from build123d import *

# Parameters (mm, degrees)
SKETCH1_W                       = 49.784
SKETCH1_H                       = 35.56
BOSS_EXTRUDE1_DEPTH             = 50.8
M4X0_7_TAPPED_HOLE1_AT_2_COUNT  = 2
M4X0_7_TAPPED_HOLE1_AT_2_PITCH  = 30
M4X0_7_TAPPED_HOLE1_AT_3_COUNT  = 2
M4X0_7_TAPPED_HOLE1_AT_3_PITCH  = 18
M4X0_7_TAPPED_HOLE1_AT_4_COUNT  = 2
M4X0_7_TAPPED_HOLE1_AT_4_PITCH  = 24
CUT_EXTRUDE2_DEPTH              = 0.508
MIRROR2_START                   = -17.78
MIRROR2_DEPTH                   = 0.508
M5X0_8_TAPPED_HOLE1_D           = 4.2
M5X0_8_TAPPED_HOLE1_DEPTH       = 12.192
M5X0_8_TAPPED_HOLE1_CSINK_D     = 6
M5X0_8_TAPPED_HOLE1_CSINK_ANGLE = 90
M5X0_8_TAPPED_HOLE1_TIP         = 1.2618073


# Read off the part's stored shape, not the designer's step: Mirror2
with BuildPart() as part:
    # Sketch1 → Boss-Extrude1 (new body)
    with BuildSketch(Plane.YZ):
        Rectangle(SKETCH1_W, SKETCH1_H)
    extrude(amount=BOSS_EXTRUDE1_DEPTH)

    # Sketch3 → M4x0.7 Tapped Hole1 (revolve, cut)
    with BuildSketch(Plane(origin=(13.4, -24.892, -9), x_dir=(0, 0, -1), z_dir=(1, 0, 0))):
        Polygon((0, 0), (0, 10.897420021), (1.65, 9.906), (1.65, 0.85), (2.5, 0), align=None)
    m4x0_7_tapped_hole1 = revolve(axis=Axis((13.4, -31.242, -9), (0, 1, 0)), mode=Mode.SUBTRACT)

    # M4x0.7 Tapped Hole1 at 2: M4x0.7 Tapped Hole1 ×2
    with Locations(*[Vector(0.8000000000000002, 0, 0.5999999999999998) * (i * M4X0_7_TAPPED_HOLE1_AT_2_PITCH) for i in range(1, M4X0_7_TAPPED_HOLE1_AT_2_COUNT)]):
        add(m4x0_7_tapped_hole1, mode=Mode.SUBTRACT)

    # M4x0.7 Tapped Hole1 at 3: M4x0.7 Tapped Hole1 ×2
    with Locations(*[(0, 0, i * M4X0_7_TAPPED_HOLE1_AT_3_PITCH) for i in range(1, M4X0_7_TAPPED_HOLE1_AT_3_COUNT)]):
        add(m4x0_7_tapped_hole1, mode=Mode.SUBTRACT)

    # M4x0.7 Tapped Hole1 at 4: M4x0.7 Tapped Hole1 ×2
    with Locations(*[(i * M4X0_7_TAPPED_HOLE1_AT_4_PITCH, 0, 0) for i in range(1, M4X0_7_TAPPED_HOLE1_AT_4_COUNT)]):
        add(m4x0_7_tapped_hole1, mode=Mode.SUBTRACT)

    # Mirror1: M4x0.7 Tapped Hole1 across plane
    add(m4x0_7_tapped_hole1.mirror(Plane.ZX), mode=Mode.SUBTRACT)

    # Mirror1 copy 1 sketch → Mirror1 copy 1 (revolve, cut)
    with BuildSketch(Plane(origin=(37.4, 24.892, 9), x_dir=(0, 0, -1), z_dir=(1, 0, 0))):
        Polygon((0, 0), (0, -10.897420021), (1.65, -9.906), (1.65, -0.85), (2.5, 0), align=None)
    revolve(axis=Axis((37.4, 31.242, 9), (0, 1, 0)), mode=Mode.SUBTRACT)

    # Mirror1 copy 2 sketch → Mirror1 copy 2 (revolve, cut)
    with BuildSketch(Plane(origin=(13.4, 24.892, 9), x_dir=(0, 0, -1), z_dir=(1, 0, 0))):
        Polygon((0, 0), (0, -10.897420021), (1.65, -9.906), (1.65, -0.85), (2.5, 0), align=None)
    revolve(axis=Axis((13.4, 31.242, 9), (0, 1, 0)), mode=Mode.SUBTRACT)

    # Mirror1 copy 3 sketch → Mirror1 copy 3 (revolve, cut)
    with BuildSketch(Plane(origin=(37.4, 24.892, -9), x_dir=(0, 0, -1), z_dir=(1, 0, 0))):
        Polygon((0, 0), (0, -10.897420021), (1.65, -9.906), (1.65, -0.85), (2.5, 0), align=None)
    revolve(axis=Axis((37.4, 31.242, -9), (0, 1, 0)), mode=Mode.SUBTRACT)

    # Sketch5 → Cut-Revolve1 (revolve, cut)
    with BuildSketch(Plane(origin=(0, 0, 0), x_dir=(-1, 0, 0), z_dir=(0, 1, 0))):
        Polygon((-25.4, 17.78), (-25.4, 13.964535069), (-31.75, 17.78), align=None)
    revolve(axis=Axis((25.4, 0, 17.78), (0, 0, -1)), mode=Mode.SUBTRACT)

    # Sketch9 → Cut-Extrude2 (cut)
    with BuildSketch(Plane(origin=(0, 0, -17.78), x_dir=(1, 0, 0), z_dir=(0, 0, -1))):
        with BuildLine():
            Line((25.4, 12.7), (31.75, 12.7))
            ThreePointArc((31.75, 12.7), (34.925, 15.875), (38.1, 12.7))
            Line((38.1, 12.7), (38.1, 6.35))
            Line((38.1, 6.35), (50.8, 6.35))
            Line((50.8, 6.35), (50.8, 0))
            Line((50.8, 0), (25.4, 0))
            Line((25.4, 0), (25.4, 12.7))
        make_face()
    extrude(amount=-CUT_EXTRUDE2_DEPTH, mode=Mode.SUBTRACT)

    # Mirror2 outline → Mirror2 (cut)
    with BuildSketch(Plane.XY.offset(MIRROR2_START)):
        with BuildLine():
            Line((38.1, 6.35), (38.1, 12.7))
            ThreePointArc((38.1, 12.7), (34.925, 15.875), (31.75, 12.7))
            Line((31.75, 12.7), (19.05, 12.7))
            ThreePointArc((19.05, 12.7), (15.875, 15.875), (12.7, 12.7))
            Line((12.7, 12.7), (12.7, 6.35))
            Line((12.7, 6.35), (0, 6.35))
            Line((0, 6.35), (0, -6.35))
            Line((0, -6.35), (12.7, -6.35))
            Line((12.7, -6.35), (12.7, -12.7))
            ThreePointArc((12.7, -12.7), (15.875, -15.875), (19.05, -12.7))
            Line((19.05, -12.7), (25.4, -12.7))
            Line((25.4, -12.7), (25.4, 0))
            Line((25.4, 0), (50.8, 0))
            Line((50.8, 0), (50.8, 6.35))
            Line((50.8, 6.35), (38.1, 6.35))
        make_face()
    extrude(amount=MIRROR2_DEPTH, mode=Mode.SUBTRACT)

    # M5x0.8 Tapped Hole1
    with Locations(Plane(origin=(0, 0, -17.272), x_dir=(1, 0, 0), z_dir=(0, 0, -1))):
        with Locations((44.45, 0)):
            CounterSinkHole(M5X0_8_TAPPED_HOLE1_D / 2, M5X0_8_TAPPED_HOLE1_CSINK_D / 2, depth=M5X0_8_TAPPED_HOLE1_DEPTH, counter_sink_angle=M5X0_8_TAPPED_HOLE1_CSINK_ANGLE)
            with Locations((0, 0, -(M5X0_8_TAPPED_HOLE1_DEPTH + M5X0_8_TAPPED_HOLE1_TIP / 2))):  # 118° drill point
                Cone(0, M5X0_8_TAPPED_HOLE1_D / 2, M5X0_8_TAPPED_HOLE1_TIP, mode=Mode.SUBTRACT)


solid = part.part
Geometry: final body of the model. Coordinates: model frame, mm. A direction names the side the tool comes from. Coordinates: 2 decimals unless noted, no trailing zeros. Return JSON: item names as keys, results as strings.
Item 1: Line query: L1, parallel to X at y = 22, z = -9; L2, parallel to Z at x = 37.4, y = 22; L3, parallel to Z at x = 13.5, y = -0.5. Output: solid intervals per line, ascending.
Completed:
{"L1": "x = 0 to 11.75, 15.05 to 35.75, 39.05 to 50.8", "L2": "z = -17.78 to -10.65, -7.35 to 7.35, 10.65 to 17.78", "L3": "z = -17.27 to 17.78"}
Item 2: Pin query (flat end, axial travel): pin 1 Ø5 at (x, y) = (45.5, 0) entering from -Z; pin 2 Ø2.5 at (x, z) = (13.4, -9) entering from +Y; pin 3 Ø2 at (x, z) = (13.4, -9) entering from +Y. Return the tip coordinate at first contact, or that it passes through.
Completed:
{"pin 1": "stops at z = -17.27", "pin 2": "stops at y = 14.75", "pin 3": "stops at y = 14.6"}
Item 3: Reachability of faces 4 (the face through (15, 19.6, -8.6)), 5 (the face through (34.855, -15.874, -17.53)), 6 (the face through (38.4, -19.58, 10.31)) from +Z, -Z, +X, -X, +Y, -Y: full face, straight path, thin tool, end or side. Return the list, or none.
Completed:
{"face 4": "+Y", "face 5": "-Z", "face 6": "-Y"}
Item 4: Pull-direction query (Z, two-part tool) for faces 1 (the face through (13.314, 14.167, 8.727)), 2 (the face through (15.945, 15.874, -17.53)), 3 (the face through (44.086, -0.016, -4.037)); classes: +Z half, -Z half, draft (parallel to the pull), parting line (faces both ways), or undercut.
Completed:
{"face 1": "undercut", "face 2": "draft", "face 3": "-Z half"}
